Can you work these out from the model? Positions are in its coordinate system, mm. A direction names the side the tool comes from. Coordinates: 2 decimals unless noted, no trailing zeros. Write each loop counter-clockwise with the first axis right and the second up, starting at its lowest first coordinate (ties: lowest second). Pieces come first, ordered by that corner, then holes. Notation, with made-up numbers: (-17, 7.5) -> (-9, 7.5) arc R13 cw to (-9, 12.5) -> close; hole circle Ø9 at (42, 84.5). An arc over 180 degrees is marked (long way). Answer as CSV lines item,"result". Start each with the question number.
```python
from build123d import *

# Parameters (mm, degrees)
BOSS_EXTRUDE2_DEPTH = 1


with BuildPart() as part:
    # Sketch2 → Boss-Extrude2 (new body)
    with BuildSketch(Plane.XY):
        with BuildLine():
            Line((-21, 21.487770019), (-17.25, 21.487770019))
            Line((-17.25, 21.487770019), (-17.25, 11.487770019))
            ThreePointArc((-17.25, 11.487770019), (-15.155, 9.392770019), (-13.06, 11.487770019))
            Line((-13.06, 11.487770019), (-13.06, 21.487770019))
            Line((-13.06, 21.487770019), (-10.56, 21.487770019))
            Line((-10.56, 21.487770019), (-10.56, 11.487770019))
            ThreePointArc((-10.56, 11.487770019), (-5, 5.927770019), (0.56, 11.487770019))
            Line((0.56, 11.487770019), (0.56, 21.487770019))
            Line((0.56, 21.487770019), (3.06, 21.487770019))
            Line((3.06, 21.487770019), (3.06, 11.487770019))
            ThreePointArc((3.06, 11.487770019), (5.155, 9.392770019), (7.25, 11.487770019))
            Line((7.25, 11.487770019), (7.25, 21.487770019))
            Line((7.25, 21.487770019), (11, 21.487770019))
            Line((11, 21.487770019), (11, 11.487770019))
            ThreePointArc((11, 11.487770019), (5.966787544, 3.86706946), (-2.220289758, -0.18016044))
            ThreePointArc((-2.220289758, -0.18016044), (-3.139034242, -0.72968283), (-3.5, -1.737536988))
            Line((-3.5, -1.737536988), (-3.5, -10.384166662))
            Line((-3.5, -10.384166662), (-6.5, -10.384166662))
            Line((-6.5, -10.384166662), (-6.5, -1.737536988))
            ThreePointArc((-6.5, -1.737536988), (-6.860965758, -0.72968283), (-7.779710242, -0.18016044))
            ThreePointArc((-7.779710242, -0.18016044), (-15.966787544, 3.86706946), (-21, 11.487770019))
            Line((-21, 11.487770019), (-21, 21.487770019))
        make_face()
    extrude(amount=BOSS_EXTRUDE2_DEPTH)


solid = part.part
```
Q1. Imagine slicing it at A-A (y = 19). Write out the boundary of the cut face in (x, z), then the cut area to 3 significant figures.
Q2. I need wall thicknesses on L1, parallel to X at y = 16.5, z = 0.3; L2, parallel to X at y = -5, z = 0.15; L3, parallel to X at y = 8.5, z = 0.9. Which ranges of each line are inside material? Lowest first, please.
Q3. If we mould it in two halves opening along X, with no side actions, what happens to faces 1 (the face through (-6.5, -6.1, 0.5)), 2 (the face through (-5.12, 5.93, 0.49)), 3 (the face through (9.1, 21.488, 0.5))? For each: released by +X, released by -X, zero draft, split by the parting line, or undercut.
Q4. Imagine slicing it at D-D (x = -5). Write out the boundary of the cut face in (y, z).
Q5. Which directions (+Z, -Z, +X, -X, +Y, -Y) give clear straight access to the entire face, cutting with the end or side of a thin tool? Please do faces 4 (the face through (-5, -10.384, 0.5)), 5 (the face through (3.06, 16.6, 0.5)).
Q6. Imagine slicing it at C-C (y = 8.5). Write out the boundary of the cut face in (x, z), then the cut area to 3 significant figures.
Entries:
1,outline,"(-21, 0) -> (-17.25, 0) -> (-17.25, 1) -> (-21, 1) -> close; (-13.06, 0) -> (-10.56, 0) -> (-10.56, 1) -> (-13.06, 1) -> close; (0.56, 0) -> (3.06, 0) -> (3.06, 1) -> (0.56, 1) -> close; (7.25, 0) -> (11, 0) -> (11, 1) -> (7.25, 1) -> close"
1,area,"12.5 mm2"
2,L1,"-21 to -17.25, -13.06 to -10.56, 0.56 to 3.06, 7.25 to 11"
2,L2,"-6.5 to -3.5"
2,L3,"-19.69 to -9.69, -0.31 to 9.69"
3,face 1,"released by -X"
3,face 2,"undercut"
3,face 3,"zero draft"
4,outline,"(-10.38, 0) -> (5.93, 0) -> (5.93, 1) -> (-10.38, 1) -> close"
5,face 4,"+Z, -Z, +X, -X, -Y"
5,face 5,"+Z, -Z, +Y"
6,outline,"(-19.69, 0) -> (-9.69, 0) -> (-9.69, 1) -> (-19.69, 1) -> close; (-0.31, 0) -> (9.69, 0) -> (9.69, 1) -> (-0.31, 1) -> close"
6,area,"20.0 mm2"
